Read the model definition and answer for the solid it produces. Units are mm, in the model's axes. A direction names the side the tool comes from. Coordinates: 2 decimals unless noted, no trailing zeros. Loops run counter-clockwise (first coordinate to the right, second up) from the corner with the lowest first, then second, coordinate; pieces in that order, holes last. Notation, with made-up numbers: (61.25, 74.5) -> (83.25, 74.5) arc R8 ccw to (83.25, 81.5) -> close; hole circle Ø10 at (56.25, 27.5). An arc over 180 degrees is marked (long way). Answer as a JSON object with one key per item and string values. Group by question number.
Q1. For faces 4 (the flat face through (-4, 9.565, 5)), 5 (the flat face through (3, 0, 4.5)), 6 (the flat face through (-4, -6.435, 4)), 7 (the flat face through (0.812, 3, 5)), determine the directions among +Z, -Z, +X, -X, +Y, -Y from which every point of the face is accessible in a straight line to the end or side of a thin tool.
Q2. The part is cut by section B-B on z = 5. Write down the section's boundary in (x, y), and give its area (3 significant figures).
Q3. Determine the mould class of faces 1 (the flat face through (3, 2, 6.5)), 2 (the flat face through (0, 2, 2.5)), 3 (the cylindrical face through (-19.59, 9.99, 1.23)) for opening direction Z: released by +Z, released by -Z, zero draft, split by the parting line, or undercut.
Q4. Each of these flat-tipped pins is pushed along its axis until it touches: P1, Ø2.5, axis at x = -14.19, y = 1.57, coming from the +Z side; P2, Ø1.2, axis at x = -2.5, z = 5, coming from the -Y side; P3, Ø2.5, axis at x = -3.5, y = 4, coming from the -Z side; P4, Ø1.2, axis at x = 2.5, z = 4, coming from the +Y side. Where does it stop, or does it pass through?
Q5. The part is cut by section C-C on z = 1.5. Write down the section's boundary in (x, y).
Q6. Straight lines are drawn through the part: line 1 along Z through (x, y) = (5.5, -5.25); line 2 along X through (y, z) = (-2.75, 5.75); line 3 along Z through (x, y) = (15.5, -1.75). For each, find the intervals that lie inside material, in ascending order. Write a range as [from, to].
Q7. The part is cut by section D-D on x = -17.5. Write down the section's boundary in (y, z), and give its area (3 significant figures).
Q8. The part is cut by section A-A on y = 6. Write down the section's boundary in (x, z), and give its area (3 significant figures).
from build123d import *

# Parameters (mm, degrees)
F0_R     = 2.25
F1_DEPTH = 2.5
F2_W     = 5
F2_H     = 3
F3_DEPTH = 2
F4_W     = 5
F4_H     = 13
F4_H_2   = 16
F4_H_3   = 3
F5_DEPTH = 2
F2_R     = 0.5
F6_DEPTH = 0.7
F6_TAPER = 25


with BuildPart() as f1:
    # F0 (on Top) → F1 (new body)
    with BuildSketch(Plane.XY):
        with BuildLine():
            Line((17.8120516539, 10.5652021154), (-18.1879483461, 10.5652021154))
            ThreePointArc((-18.1879483461, 10.5652021154), (-19.6021619085, 9.9794156778), (-20.1879483461, 8.5652021154))
            Line((-20.1879483461, 8.5652021154), (-20.1879483461, -5.4347978846))
            ThreePointArc((-20.1879483461, -5.4347978846), (-19.6021619085, -6.849011447), (-18.1879483461, -7.4347978846))
            Line((-18.1879483461, -7.4347978846), (17.8120516539, -7.4347978846))
            ThreePointArc((17.8120516539, -7.4347978846), (19.2262652162, -6.849011447), (19.8120516539, -5.4347978846))
            Line((19.8120516539, -5.4347978846), (19.8120516539, 8.5652021154))
            ThreePointArc((19.8120516539, 8.5652021154), (19.2262652162, 9.9794156778), (17.8120516539, 10.5652021154))
        make_face()
        with Locations((-14.1879483461, 1.5652021154)):
            Circle(F0_R, mode=Mode.SUBTRACT)
        with Locations((13.8120516539, 1.5652021154)):
            Circle(F0_R, mode=Mode.SUBTRACT)
    extrude(amount=F1_DEPTH)

    # F2 (on face) → F3 (join)
    with BuildSketch(Plane.XY.offset(2.5)):
        with Locations((-3.6879483461, -4.9347978846)):
            Rectangle(F2_W, F2_H)
        with Locations((3.3120516539, 8.0652021154)):
            Rectangle(F2_W, F2_H)
    extrude(amount=F3_DEPTH)

    # F4 (on face) → F5 (join)
    with BuildSketch(Plane.XY.offset(4.5)):
        with Locations((-3.6879483461, 3.0652021154)):
            Rectangle(F4_W, F4_H)
        with Locations((3.3120516539, 1.5652021154)):
            Rectangle(F4_W, F4_H_2)
        with Locations((-3.6879483461, -4.9347978846)):
            Rectangle(F4_W, F4_H_3)
    extrude(amount=F5_DEPTH)

    # F2 (on face) → F6 (join)
    with BuildSketch(Plane.XY.offset(2.5)):
        with Locations((-3.6879483461, 8.0652021154)):
            Circle(F2_R)
        with Locations((3.3120516539, -4.9347978846)):
            Circle(F2_R)
    extrude(amount=F6_DEPTH, taper=F6_TAPER)


solid = f1.part
Final values:
{
 "1": {"face 4": "+Z, +X, -X, +Y", "face 5": "+X, -Y", "face 6": "+Z, +X, -X, -Y", "face 7": "+Z, +Y, -Y"},
 "2": {"outline": "(-6.19, -6.43) -> (-1.19, -6.43) -> (-1.19, 9.57) -> (-6.19, 9.57) -> close; (0.81, -6.43) -> (5.81, -6.43) -> (5.81, 9.57) -> (0.81, 9.57) -> close", "area": "160 mm2"},
 "3": {"face 1": "released by +Z", "face 2": "undercut", "face 3": "zero draft"},
 "4": {"P1": "passes through", "P2": "stops at y = -6.43", "P3": "stops at z = 0", "P4": "stops at y = 9.57"},
 "5": {"outline": "(-20.19, -5.43) arc R2 ccw to (-18.19, -7.43) -> (17.81, -7.43) arc R2 ccw to (19.81, -5.43) -> (19.81, 8.57) arc R2 ccw to (17.81, 10.57) -> (-18.19, 10.57) arc R2 ccw to (-20.19, 8.57) -> close; hole circle Ø4.5 at (-14.19, 1.57); hole circle Ø4.5 at (13.81, 1.57)"},
 "6": {"line 1": "z = [0, 2.5], [4.5, 6.5]", "line 2": "x = [-6.19, -1.19], [0.81, 5.81]", "line 3": "z = [0, 2.5]"},
 "7": {"outline": "(-7.43, 0) -> (10.57, 0) -> (10.57, 2.5) -> (-7.43, 2.5) -> close", "area": "45.0 mm2"},
 "8": {"outline": "(-20.19, 0) -> (19.81, 0) -> (19.81, 2.5) -> (-20.19, 2.5) -> close; (-6.19, 4.5) -> (-1.19, 4.5) -> (-1.19, 6.5) -> (-6.19, 6.5) -> close; (0.81, 4.5) -> (5.81, 4.5) -> (5.81, 6.5) -> (0.81, 6.5) -> close", "area": "120 mm2"}
}
